Verification items for this drawing (mm, ordinates from the low corner). A direction names the side the tool comes from. Coordinates: 2 decimals unless noted, no trailing zeros. Write each loop counter-clockwise with the first axis right and the second up, starting at its lowest first coordinate (ties: lowest second). Pieces come first, ordered by that corner, then holes. Notation, with made-up numbers: (-27, -23) -> (21, -23) arc R15 ccw to (21, -10) -> close; hole circle Ø4 at (43, 2). An arc over 180 degrees is marked (long way). Put each result on its own line as item: value. Start each with the question number.
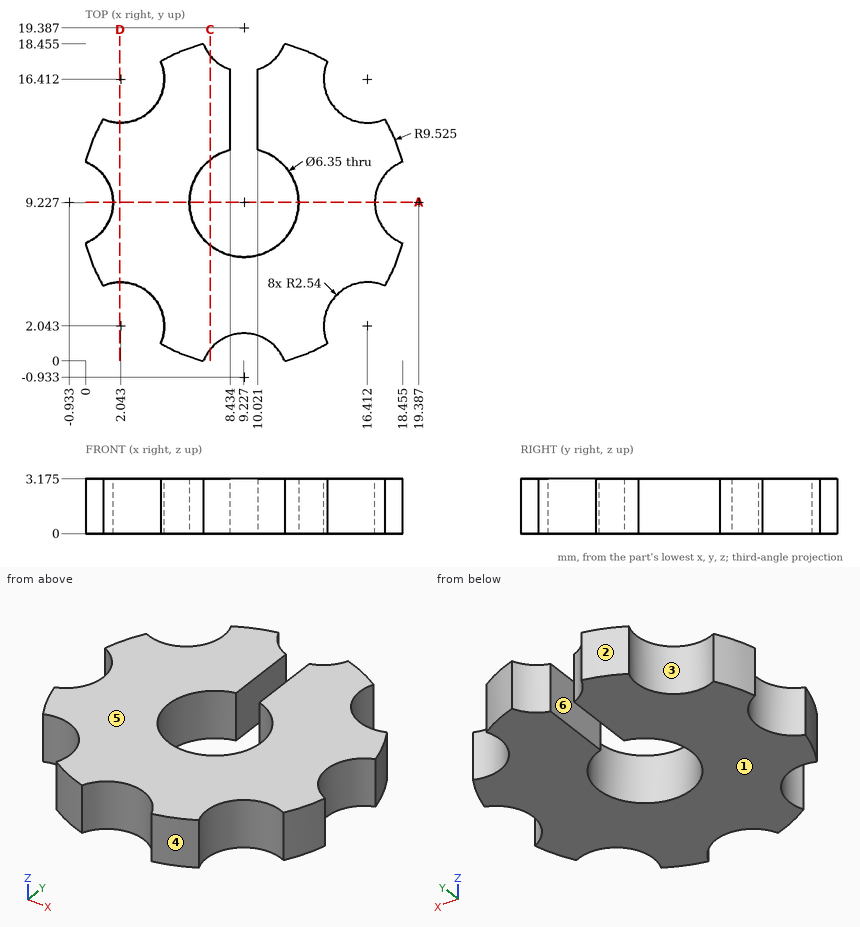
Item 1: Scan lines: line 1 along X through (y, z) = (2, 1.6); line 2 along X through (y, z) = (7.75, 2.85) (1 decimal); line 3 along Y through (x, z) = (7.5, 0.7) (1 decimal). Record each from-to range of solid material in increasing order. Write a range as [from, to].
Item 2: Section check A-A, the plane y = 9.25. Enter the section's corners in (x, z) (1 decimal).
Item 3: Access from +Z, -Z, +X, -X, +Y, -Y to the whole of each face (thin tool, end or side, straight path). Record for the marked faces 5 and 6.
Item 4: Section check D-D, the plane x = 2. Enter the section's corners in (y, z) (1 decimal).
Item 5: Go/stop test with flat-tipped pins: P1, Ø2, axis at x = 10, y = 11, coming from the +Z side; P2, Ø1, axis at x = 12.5, z = 1.5, coming from the -Y side (1 decimal). Record where each tip stops, or that it passes through.
Item 6: Section check C-C, the plane x = 7.25. Enter the section's corners in (y, z) (1 decimal).
Item 7: Mould release check, pull along X, two halves, no side actions. Record for the marked faces 1, 2, 3 and 4: released by +X, released by -X, zero draft, split by the parting line, or undercut.
From the geometry:
1. line 1: [4.58, 13.87]
1. line 2: [1.1, 6.4], [12, 17.3]
1. line 3: [0.9, 6.6], [11.9, 17.5]
2. outline: (1.6, 0) -> (6.1, 0) -> (6.1, 3.2) -> (1.6, 3.2) -> close; (12.4, 0) -> (16.8, 0) -> (16.8, 3.2) -> (12.4, 3.2) -> close
3. face 5: +Z, +X, -X, +Y, -Y
3. face 6: +Z, -Z, +Y
4. outline: (4.6, 0) -> (13.9, 0) -> (13.9, 3.2) -> (4.6, 3.2) -> close
5. P1: through
5. P2: y = 0.1
6. outline: (0.7, 0) -> (6.7, 0) -> (6.7, 3.2) -> (0.7, 3.2) -> close; (11.7, 0) -> (17.8, 0) -> (17.8, 3.2) -> (11.7, 3.2) -> close
7. face 1: zero draft
7. face 2: released by -X
7. face 3: undercut
7. face 4: released by +X
